Read the model definition and answer for the solid it produces. Units are mm, in the model's axes. A direction names the side the tool comes from. Coordinates: 2 decimals unless noted, no trailing zeros. Order: outer loops, then holes, each group sorted by start corner. A loop starts at its lowest first (then second) coordinate and runs counter-clockwise, first axis right, second up. Notation, with made-up numbers: M 5.25,45.5 L 36.25,45.5 A11 ccw 36.25,53.5 Z; hole C 63,28 d11. An arc over 180 degrees is marked long. One line per question, with ' | ' between items. Start each with the question number.
1) Find section A-A, the plane z = 0. Write down the section's boundary in (x, y).
2) A tool of negligible diameter and unlimited length cuts with its end or side. For faces 1 (the face through (-8, 0, 8)), 2 (the face through (-20.543, -13.102, 6.905)), from which of +Z, -Z, +X, -X, +Y, -Y can it reach the whole face along a straight path? Write none if from no direction.
3) Given P1, Ø7.5, axis at y = -17, z = 6, coming from the +X side; P2, Ø2, axis at y = -4.56, z = 0, coming from the +X side; P3, Ø4, axis at x = -6.92, z = -13.31, coming from the -Y side, each flat-ended and moving along its own axis, determine where each tip first touches the part or whether it passes through.
4) Find section C-C, the plane y = 1.5. Write down the section's boundary in (x, z), plus the area to 3 significant figures.
5) Find section D-D, the plane z = 6. Write down the section's boundary in (x, y), plus the area to 3 significant figures.
6) Consider probe 1 along Y at (x, z) = (-20.3, 0); probe 2 along X at (y, z) = (1.5, 0); probe 3 along Y at (x, z) = (-20.05, 8.06). Determine where each line is inside the solid, lowest interval first.
7) The mould has two halves that part along X. Classify faces 3 (the face through (-6.542, 1.479, 12.475)), 4 (the face through (-22.571, -11, 0)), 5 (the face through (19.185, 1.479, 0.422)), 6 (the face through (-19, -7, -19.19)): +X half, -X half, draft (parallel to the pull), parting line (faces both ways), or undercut.
8) Find section B-B, the plane x = -3.5. Write down the section's boundary in (y, z).
from build123d import *

# Parameters (mm, degrees)
SKETCH1_R           = 10.25
SKETCH1_R_2         = 1.5
BOSS_EXTRUDE3_DEPTH = 3
SKETCH2_W           = 4
SKETCH2_H           = 38.38
BOSS_EXTRUDE4_DEPTH = 25.4
SKETCH3_R           = 1.25
CUT_EXTRUDE2_DEPTH  = 25.4


with BuildPart() as part:
    # Sketch1 → Boss-Extrude3 (new body)
    with BuildSketch(Plane(origin=(0, 0, 0), x_dir=(1, 0, 0), z_dir=(0, 1, 0))):
        with BuildLine():
            Line((-22.571326258, -19.19), (0, -19.19))
            ThreePointArc((0, -19.19), (19.19, 0), (0, 19.19))
            Line((0, 19.19), (-22.571326258, 19.19))
            Line((-22.571326258, 19.19), (-22.571326258, -19.19))
        make_face()
        with Locations(Location((0, 0, 0), (0, 0, 270))):
            Circle(SKETCH1_R, mode=Mode.SUBTRACT)
        with Locations(Location((-6.923626209, 13.306517204, 0), (0, 0, 270))):
            Circle(SKETCH1_R_2, mode=Mode.SUBTRACT)
        with Locations(Location((-8.029460065, -12.669955448, 0), (0, 0, 270))):
            Circle(SKETCH1_R_2, mode=Mode.SUBTRACT)
        with Locations(Location((14.988772764, -0.580250843, 0), (0, 0, 270))):
            Circle(SKETCH1_R_2, mode=Mode.SUBTRACT)
    extrude(amount=BOSS_EXTRUDE3_DEPTH)

    # Sketch2 → Boss-Extrude4 (add)
    with BuildSketch(Plane.XZ):
        with Locations((-20.571326258, 0)):
            Rectangle(SKETCH2_W, SKETCH2_H)
    extrude(amount=BOSS_EXTRUDE4_DEPTH)

    # Sketch3 → Cut-Extrude2 (cut)
    with BuildSketch(Plane(origin=(-18.571326258, 0, 0), x_dir=(0, 0, -1), z_dir=(1, 0, 0))):
        with Locations((0, -4.563544693)):
            Circle(SKETCH3_R)
        with Locations((-8.06, -12.623544693)):
            Circle(SKETCH3_R)
        with Locations((0, -20.683544693)):
            Circle(SKETCH3_R)
        with Locations((8.06, -12.623544693)):
            Circle(SKETCH3_R)
    extrude(amount=-CUT_EXTRUDE2_DEPTH, mode=Mode.SUBTRACT)


solid = part.part
Report:
1) outline: M -22.57,-25.4 L -18.57,-25.4 L -18.57,-21.93 L -22.57,-21.93 Z; M -22.57,-19.43 L -18.57,-19.43 L -18.57,-5.81 L -22.57,-5.81 Z; M -22.57,-3.31 L -18.57,-3.31 L -18.57,0 L -10.25,0 L -10.25,3 L -22.57,3 Z; M 10.25,0 L 13.61,0 L 13.61,3 L 10.25,3 Z; M 16.37,0 L 19.19,0 L 19.19,3 L 16.37,3 Z
2) face 1: +Z, -Z, +X, -Y | face 2: +X, -X
3) P1: stops at x = -18.57 | P2: passes through | P3: stops at y = 0
4) outline: M -22.57,-19.19 L 0,-19.19 A19.19 ccw 0,19.19 L -22.57,19.19 Z; hole C 0,0 d20.5; hole C -8.03,12.67 d3; hole C -6.92,-13.31 d3; hole C 14.99,0.58 d3 | area: 1,090 mm^2
5) outline: M -22.57,-25.4 L -18.57,-25.4 L -18.57,0 L -8.31,0 L -8.31,3 L -22.57,3 Z; M 8.31,0 L 18.23,0 L 18.23,3 L 8.31,3 Z | area: 174 mm^2
6) probe 1: y = -25.4 to -21.93, -19.43 to -5.81, -3.31 to 3 | probe 2: x = -22.57 to -10.25, 10.25 to 13.61, 16.37 to 19.19 | probe 3: y = -25.4 to -13.87, -11.37 to 3
7) face 3: undercut | face 4: -X half | face 5: +X half | face 6: draft
8) outline: M 0,-19.19 L 3,-19.19 L 3,-9.63 L 0,-9.63 Z; M 0,9.63 L 3,9.63 L 3,19.19 L 0,19.19 Z
